```python
from build123d import *

# Parameters (mm, degrees)
SKETCH_W        = 51
SKETCH_H        = 33.5
PAD_DEPTH       = 85
SKETCH001_W     = 27
SKETCH001_H     = 9
SKETCH001_W_2   = 44
SKETCH001_H_2   = 13.5
POCKET_DEPTH    = 85
FILLET_R        = 16
FILLET001_R     = 1.5
SKETCH002_R     = 5
POCKET001_DEPTH = 17
SKETCH003_R     = 3
POCKET002_DEPTH = 3.001
CHAMFER_SIZE    = 1.75
FILLET002_R     = 1
FILLET003_R     = 1


with BuildPart() as part:
    # Sketch → Pad (new body)
    with BuildSketch(Plane.XY):
        Rectangle(SKETCH_W, SKETCH_H)
    extrude(amount=PAD_DEPTH)

    # Sketch001 (on Face6 of Pad) → Pocket (cut)
    with BuildSketch(Plane.XY.offset(85)):
        with Locations((0, 8.25)):
            Rectangle(SKETCH001_W, SKETCH001_H)
        with Locations((0, -7)):
            Rectangle(SKETCH001_W_2, SKETCH001_H_2)
    extrude(amount=-POCKET_DEPTH, mode=Mode.SUBTRACT)

    # Fillet
    fillet_edges = [part.edges().sort_by_distance(p)[0] for p in [
        (25.5, 16.75, 42.5),
        (-25.5, 16.75, 42.5),
    ]]
    fillet(fillet_edges, radius=FILLET_R)

    # Fillet001
    fillet001_edges = [part.edges().sort_by_distance(p)[0] for p in [
        (20.813708, 12.063708, 85),
        (25.5, -8, 85),
        (0, 16.75, 85),
        (-20.813708, 12.063708, 85),
        (-25.5, -8, 85),
    ]]
    fillet(fillet001_edges, radius=FILLET001_R)

    # Sketch002 (on Face7 of Fillet001) → Pocket001 (cut)
    with BuildSketch(Plane(origin=(0, 16.75, 0), x_dir=(-1, 0, 0), z_dir=(0, 1, 0))):
        with Locations((0, 70)):
            Circle(SKETCH002_R)
        with Locations((0, 15)):
            Circle(SKETCH002_R)
    extrude(amount=-POCKET001_DEPTH, mode=Mode.SUBTRACT)

    # Sketch003 (on Face13 of Pocket001) → Pocket002 (cut, through all)
    with BuildSketch(Plane(origin=(0, -13.75, 0), x_dir=(-1, 0, 0), z_dir=(0, 1, 0))):
        with Locations((0, 70)):
            Circle(SKETCH003_R)
        with Locations((0, 15)):
            Circle(SKETCH003_R)
    extrude(amount=-POCKET002_DEPTH, mode=Mode.SUBTRACT)

    # Chamfer
    chamfer_edges = [part.edges().sort_by_distance(p)[0] for p in [
        (3, -13.75, 15),
        (3, -13.75, 70),
    ]]
    chamfer(chamfer_edges, length=CHAMFER_SIZE)

    # Fillet002
    fillet002_edges = [part.edges().sort_by_distance(p)[0] for p in [
        (20.813708, 12.063708, 0),
        (-20.813708, 12.063708, 0),
    ]]
    fillet(fillet002_edges, radius=FILLET002_R)

    # Fillet003
    fillet003_edges = [part.edges().sort_by_distance(p)[0] for p in [
        (0, 3.75, 0),
        (-13.5, 8.25, 0),
        (0, 12.75, 0),
        (13.5, 8.25, 0),
        (0, -0.25, 0),
        (22, -7, 0),
        (0, -13.75, 0),
        (-22, -7, 0),
    ]]
    fillet(fillet003_edges, radius=FILLET003_R)


solid = part.part
```
The model under review builds one solid part; all positions refer to its coordinate system, in mm. A direction names the side the tool comes from. Give positions to 0.01 mm unless a question says otherwise; leave off trailing zeros. Write each loop counter-clockwise with the first axis right and the second up, starting at its lowest first coordinate (ties: lowest second). Pieces come first, ordered by that corner, then holes. Notation, with made-up numbers: (41, 66.25) -> (66, 66.25) arc R8 ccw to (66, 76.25) -> close; hole circle Ø9 at (76, -34.75). An arc over 180 degrees is marked (long way). Answer in a Markdown table with one row per item.
1) Add section C-C on x = -6. State the section outline as (y, z) points.
Worked answers:
| item | result |
|---|---|
| outline | (-16.75, 0) -> (-14.75, 0) arc R1 ccw to (-13.75, 1) -> (-13.75, 85) -> (-16.75, 85) -> close; (-0.25, 1) arc R1 ccw to (0.75, 0) -> (2.75, 0) arc R1 ccw to (3.75, 1) -> (3.75, 85) -> (-0.25, 85) -> close; (12.75, 1) arc R1 ccw to (13.75, 0) -> (15.75, 0) arc R1 ccw to (16.75, 1) -> (16.75, 83.5) arc R1.5 ccw to (15.25, 85) -> (12.75, 85) -> close |
2) Tool access review of faces 1 (the cylindrical face through (0.65, -16.12, 67.07)), 2 (the cylindrical face through (1.08, 14.78, 10.12)), 3 (the flat face through (-22, -7, 44)): name each direction out of +Z, -Z, +X, -X, +Y, -Y from which nothing blocks a thin tool from reaching the whole face with its end or side.
Worked answers:
| item | result |
|---|---|
| face 1 | +Y, -Y |
| face 2 | +Y |
| face 3 | +Z, -Z |
3) Add section B-B on y = -10.5. State the section outline as (x, z) points.
Worked answers:
| item | result |
|---|---|
| outline | (-25.5, 1) arc R1 ccw to (-24.5, 0) -> (-23, 0) arc R1 ccw to (-22, 1) -> (-22, 85) -> (-24, 85) arc R1.5 ccw to (-25.5, 83.5) -> close; (22, 1) arc R1 ccw to (23, 0) -> (24.5, 0) arc R1 ccw to (25.5, 1) -> (25.5, 83.5) arc R1.5 ccw to (24, 85) -> (22, 85) -> close |
4) For L1, parallel to Z at x = 0, y = -16; L2, parallel to Y at x = 5.5, z = 73.5; L3, parallel to X at y = -7.5, z = 8, list the stretches that pass through material, from the lowest coordinate up. Write a range as [from, to].
Worked answers:
| item | result |
|---|---|
| L1 | [0, 12], [18, 67], [73, 85] |
| L2 | [-16.75, -13.75], [-0.25, 3.75], [12.75, 16.75] |
| L3 | [-25.5, -22], [22, 25.5] |
5) Add section A-A on z = 70. State the section outline as (x, y) points.
Worked answers:
| item | result |
|---|---|
| outline | (-25.5, -16.75) -> (-3, -16.75) -> (-3, -15.5) -> (-4.75, -13.75) -> (-22, -13.75) -> (-22, -0.25) -> (-5, -0.25) -> (-5, 3.75) -> (-13.5, 3.75) -> (-13.5, 12.75) -> (-5, 12.75) -> (-5, 16.75) -> (-9.5, 16.75) arc R16 ccw to (-25.5, 0.75) -> close; (3, -16.75) -> (25.5, -16.75) -> (25.5, 0.75) arc R16 ccw to (9.5, 16.75) -> (5, 16.75) -> (5, 12.75) -> (13.5, 12.75) -> (13.5, 3.75) -> (5, 3.75) -> (5, -0.25) -> (22, -0.25) -> (22, -13.75) -> (4.75, -13.75) -> (3, -15.5) -> close |
6) Add section D-D on x = 0. Count the separate pieces of the cut face and the enclosed holes in it, plus the area to 3 significant figures.
Worked answers:
| item | result |
|---|---|
| separate pieces | 9 |
| enclosed holes | 0 |
| area | 731 mm² |
7) Mouldability with a two-part tool opening along Y and no side actions: class faces 4 (the cylindrical face through (20.689, 12.187, 42.828)), 5 (the flat face through (0, 3, 85)), 6 (the flat face through (0, 3.75, 44)) as +Y half, -Y half, draft (parallel to the pull), parting line (faces both ways), or undercut.
Worked answers:
| item | result |
|---|---|
| face 4 | +Y half |
| face 5 | draft |
| face 6 | undercut |
8) Clearance check with flat-ended pins moving along their axes: P1, Ø6, axis at y = 12.5, z = 16.5, coming from the +X side; P2, Ø6, axis at y = 6.5, z = 50.5, coming from the -X side; P3, Ø7, axis at y = 9, z = 26.5, coming from the +X side. State where each tip first meets the part, or that it passes through.
Worked answers:
| item | result |
|---|---|
| P1 | x = 22.9 |
| P2 | x = -25.26 |
| P3 | x = 24.78 |
